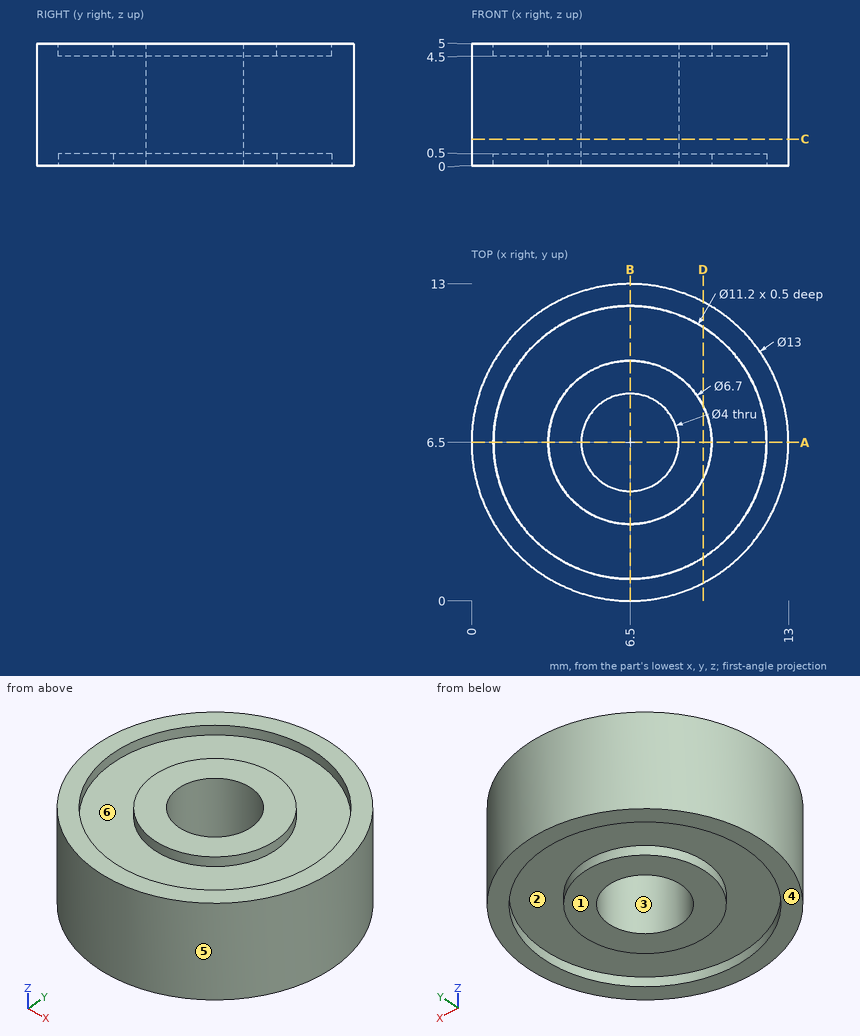
For this review, use the dimensioned drawing (mm, ordinates from the lowest corner) and the shaded views. A direction names the side the tool comes from. Round coordinates to 2 decimals unless told otherwise and drop trailing zeros. Write each loop counter-clockwise with the first axis right and the second up, starting at its lowest first coordinate (ties: lowest second). Pieces come first, ordered by that corner, then holes. Notation, with made-up numbers: (-30.75, 48) -> (22.25, 48) arc R30 cw to (22.25, 75) -> close; hole circle Ø6 at (80.5, 73.25). An arc over 180 degrees is marked (long way). Use CSV: the item, a comma, the result in double quotes.
(1) Consider section C-C, the plane z = 1.1. Give the boundary of the cut face in (x, y).
Computed values:
outline,"circle Ø13 at (6.5, 6.5); hole circle Ø4 at (6.5, 6.5)"
(2) Draft analysis for pull direction X (two halves, no side actions). For the marked faces 3, 4, 5 and 6, state which applies: +X half, -X half, draft (parallel to the pull), parting line (faces both ways), or undercut.
Computed values:
face 3,"undercut"
face 4,"draft"
face 5,"parting line"
face 6,"undercut"
(3) Clearance check with flat-ended pins moving along their axes: P1, Ø3, axis at y = 9.5, z = 4, coming from the -X side; P2, Ø3.5, axis at x = 6.5, y = 6.5, coming from the -Z side; P3, Ø2, axis at x = 3.5, z = 4, coming from the +Y side; P4, Ø1, axis at x = 2, y = 8, coming from the +Z side. State where each tip first meets the part, or that it passes through.
Computed values:
P1,"x = 0.18"
P2,"through"
P3,"y = 12.68"
P4,"z = 4.5"
(4) To check wall thickness, follow L1, parallel to Y at x = 6.5, z = 0.3; L2, parallel to X at y = 5.25, z = 0.4; L3, parallel to Y at x = 9, z = 0.3. State the ranges of each line that lie inside material, in increasing order. Write a range as [from, to].
Computed values:
L1,"[0, 0.9], [3.15, 4.5], [8.5, 9.85], [12.1, 13]"
L2,"[0.12, 1.04], [3.39, 4.94], [8.06, 9.61], [11.96, 12.88]"
L3,"[0.5, 1.49], [4.27, 8.73], [11.51, 12.5]"
(5) For the marked faces 1 and 2, list the 3-axis set-ups (+Z, -Z, +X, -X, +Y, -Y) from which the entire face can be reached by the end or side of a thin tool; tool diameter is ignored.
Computed values:
face 1,"-Z, +X, -X, +Y, -Y"
face 2,"-Z"
(6) Consider section D-D, the plane x = 9.5. Give the boundary of the cut face in (y, z), plus the area to 3 significant figures.
Computed values:
outline,"(0.73, 0) -> (1.77, 0) -> (1.77, 0.5) -> (5.01, 0.5) -> (5.01, 0) -> (7.99, 0) -> (7.99, 0.5) -> (11.23, 0.5) -> (11.23, 0) -> (12.27, 0) -> (12.27, 5) -> (11.23, 5) -> (11.23, 4.5) -> (7.99, 4.5) -> (7.99, 5) -> (5.01, 5) -> (5.01, 4.5) -> (1.77, 4.5) -> (1.77, 5) -> (0.73, 5) -> close"
area,"51.2 mm²"
(7) Consider section A-A, the plane y = 6.5. Give the boundary of the cut face in (x, z), plus the area to 3 significant figures.
Computed values:
outline,"(0, 0) -> (0.9, 0) -> (0.9, 0.5) -> (3.15, 0.5) -> (3.15, 0) -> (4.5, 0) -> (4.5, 5) -> (3.15, 5) -> (3.15, 4.5) -> (0.9, 4.5) -> (0.9, 5) -> (0, 5) -> close; (8.5, 0) -> (9.85, 0) -> (9.85, 0.5) -> (12.1, 0.5) -> (12.1, 0) -> (13, 0) -> (13, 5) -> (12.1, 5) -> (12.1, 4.5) -> (9.85, 4.5) -> (9.85, 5) -> (8.5, 5) -> close"
area,"40.5 mm²"
